Geometry check sheet. Reference: the model listing, model coordinates, mm. Give positions to 0.01 mm unless a question says otherwise; leave off trailing zeros. Order: outer loops, then holes, each group sorted by start corner. A loop starts at its lowest first (then second) coordinate and runs counter-clockwise, first axis right, second up.
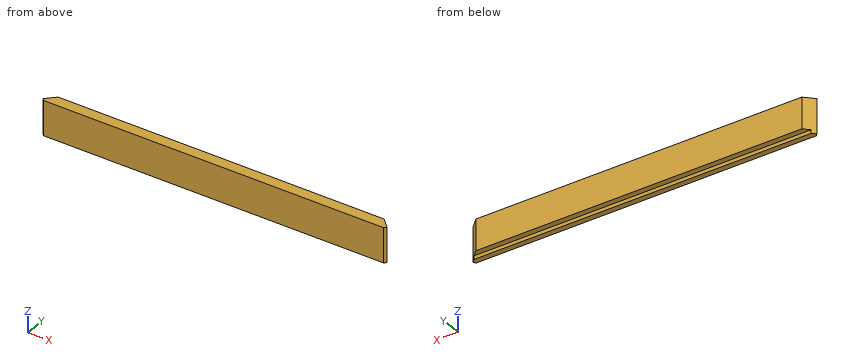
from build123d import *

# Parameters (mm, degrees)
F1_DEPTH = 60
F2_DEPTH = 6


with BuildPart() as f1:
    # F0 (on Top) → F1 (new body)
    with BuildSketch(Plane.XY):
        Polygon((0, 9.5), (0, 0), (292.9289321881, 0), (296.4644660941, 3.5355339059), (290.5, 9.5), align=None)
        Polygon((0, 19), (0, 9.5), (290.5, 9.5), (281, 19), align=None)
    extrude(amount=F1_DEPTH)

    # F0 (on Top) → F2 (cut)
    with BuildSketch(Plane.XY):
        Polygon((0, 19), (0, 9.5), (290.5, 9.5), (281, 19), align=None)
    extrude(amount=F2_DEPTH, mode=Mode.SUBTRACT)

    # F3: F1 across plane


with BuildPart() as f1_1:
    add(f1.part)
    add(f1.part.mirror(Plane.YZ))


solid = f1_1.part
Item 1: Sectioned sample at C-C (y = 13.75). Enter the section's corners in (x, z).
Reported:
outline: (-286.25, 6) - (286.25, 6) - (286.25, 60) - (-286.25, 60) - close
Item 2: Scan lines: L1, parallel to Z at x = -150, y = 12.5; L2, parallel to Y at x = -132.5, z = 4; L3, parallel to X at y = 17.25, z = 49.5. Record each from-to range of solid material in increasing order.
Reported:
L1: z = 6 to 60
L2: y = 0 to 9.5
L3: x = -282.75 to 282.75
Item 3: Sectioned sample at B-B (z = 53). Enter the section's corners in (x, y), and give its area (3 significant figures).
Reported:
outline: (-296.46, 3.54) - (-292.93, 0) - (292.93, 0) - (296.46, 3.54) - (281, 19) - (-281, 19) - close
area: 11,000 mm2
Item 4: Sectioned sample at A-A (x = 89). Enter the section's corners in (y, z), and give its area (3 significant figures).
Reported:
outline: (0, 0) - (9.5, 0) - (9.5, 6) - (19, 6) - (19, 60) - (0, 60) - close
area: 1,080 mm2
Item 5: Gauge pin test, flat ends, axial feed: pin 1 (1.8 mm diameter, centred on x = -57, z = 4.5, fed in from +Y); pin 2 (3 mm diameter, centred on x = 215, y = 14.5, fed in from -Z); pin 3 (5 mm diameter, centred on y = 5, z = 8.5, fed in from -X); pin 4 (1 mm diameter, centred on y = 9.5, z = 39.5, fed in from -X). Record the tip position at first contact, or that the pin passes through.
Reported:
pin 1: stops at y = 9.5
pin 2: stops at z = 6
pin 3: stops at x = -296.46
pin 4: stops at x = -291
